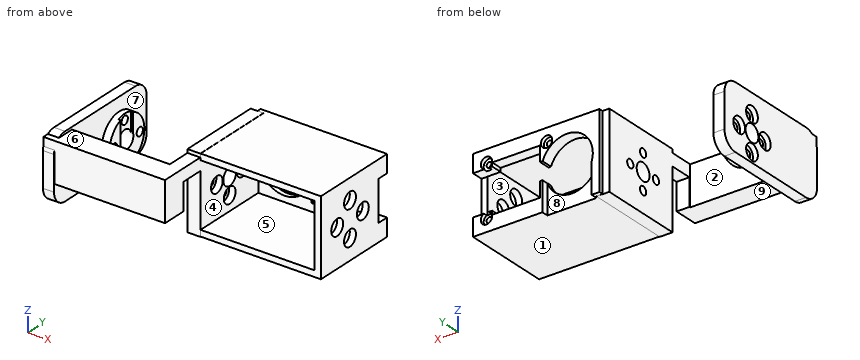
from build123d import *

# Parameters (mm, degrees)
S_PRISM1_W      = 30.9
S_PRISM1_H      = 34.5
BOSS_1_DEPTH    = 5.2
S_CYL2_R        = 9.5
BOSS_2_DEPTH    = 3.2
BOSS_3_DEPTH    = 4.5
S_BOX4_W        = 2.5
S_BOX4_H        = 36.1
BOSS_4_DEPTH    = 30.8
S_BOX5_W        = 2.5
S_BOX5_H        = 36.1
BOSS_5_DEPTH    = 30.8
S_BOX6_W        = 51.4
S_BOX6_H        = 36.1
BOSS_6_DEPTH    = 2.5
S_BOX7_W        = 51.4
S_BOX7_H        = 36.1
BOSS_7_DEPTH    = 2.5
S_BOX8_W        = 51.4
S_BOX8_H        = 4.6
BOSS_8_DEPTH    = 30.8
S_BOX9_W        = 5.2
S_BOX9_H        = 9.8
BOSS_9_DEPTH    = 5
S_BOX10_W       = 5.2
S_BOX10_H       = 10
BOSS_10_DEPTH   = 16
S_BOX11_W       = 49.45
S_BOX11_H       = 9.6
BOSS_11_DEPTH   = 16
S_HOLE12_R      = 3.5
HOLE_12_DEPTH   = 5.4
S_HOLE13_R      = 1.7
HOLE_13_DEPTH   = 5.4
S_HOLE14_R      = 1.7
HOLE_14_DEPTH   = 5.4
S_HOLE15_R      = 1.7
HOLE_15_DEPTH   = 5.4
S_HOLE16_R      = 1.7
HOLE_16_DEPTH   = 5.4
S_HOLE17_R      = 3.2
HOLE_17_DEPTH   = 2.7
S_HOLE18_R      = 3.2
HOLE_18_DEPTH   = 2.7
S_HOLE19_R      = 3.2
HOLE_19_DEPTH   = 2.7
S_HOLE20_R      = 3.2
HOLE_20_DEPTH   = 2.7
S_HOLE21_R      = 3.5
HOLE_21_DEPTH   = 7.9
S_HOLE22_R      = 1.7
HOLE_22_DEPTH   = 7.9
S_HOLE23_R      = 1.7
HOLE_23_DEPTH   = 7.9
S_HOLE24_R      = 1.7
HOLE_24_DEPTH   = 7.9
S_HOLE25_R      = 1.7
HOLE_25_DEPTH   = 7.9
S_HOLE26_R      = 3.2
HOLE_26_DEPTH   = 2.1
S_HOLE27_R      = 3.2
HOLE_27_DEPTH   = 2.1
S_HOLE28_R      = 3.2
HOLE_28_DEPTH   = 2.1
S_HOLE29_R      = 3.2
HOLE_29_DEPTH   = 2.1
S_CUT30_W       = 1
S_CUT30_H       = 6.8
POCKET_30_DEPTH = 10
S_HOLE31_R      = 10.5
HOLE_31_DEPTH   = 4.8
S_CUT32_W       = 19.5
S_CUT32_H       = 4.75
POCKET_32_DEPTH = 19.4
S_CUT33_W       = 8.3
S_CUT33_H       = 4.75
POCKET_33_DEPTH = 16.4
S_CUT34_W       = 11
S_CUT34_H       = 4.75
POCKET_34_DEPTH = 7
S_CUT35_W       = 20
S_CUT35_H       = 2.9
POCKET_35_DEPTH = 15.9
S_HOLE36_R      = 1.1
HOLE_36_DEPTH   = 4.8
S_HOLE37_R      = 2.3
HOLE_37_DEPTH   = 1.7
S_HOLE38_R      = 1.1
HOLE_38_DEPTH   = 4.8
S_HOLE39_R      = 2.3
HOLE_39_DEPTH   = 1.7
S_HOLE40_R      = 1.1
HOLE_40_DEPTH   = 4.8
S_HOLE41_R      = 2.3
HOLE_41_DEPTH   = 1.7
S_HOLE42_R      = 3.25
HOLE_42_DEPTH   = 2.7
S_HOLE43_R      = 3.25
HOLE_43_DEPTH   = 2.7
S_HOLE44_R      = 3.25
HOLE_44_DEPTH   = 2.7
S_HOLE45_R      = 3.25
HOLE_45_DEPTH   = 2.7


with BuildPart() as part:
    # S_prism1 → Boss_1 (new body)
    with BuildSketch(Plane(origin=(-15.9, 0, 0), x_dir=(0, 0, -1), z_dir=(1, 0, 0))):
        with Locations((0, 1.2)):
            Rectangle(S_PRISM1_W, S_PRISM1_H)
    extrude(amount=BOSS_1_DEPTH)

    # S_box4 → Boss_4 (add)
    with BuildSketch(Plane.XY.offset(-15.4)):
        with Locations((-11.95, 2.15)):
            Rectangle(S_BOX4_W, S_BOX4_H)
    extrude(amount=BOSS_4_DEPTH)



with BuildPart() as body_2:
    # S_cyl2 → Boss_2 (new body)
    with BuildSketch(Plane(origin=(-55.65, 0, 0), x_dir=(0, 0, -1), z_dir=(1, 0, 0))):
        Circle(S_CYL2_R)
    extrude(amount=BOSS_2_DEPTH)

    # S_prism3 → Boss_3 (add)
    with BuildSketch(Plane(origin=(-60.15, 0, 0), x_dir=(0, 0, -1), z_dir=(1, 0, 0))):
        with BuildLine():
            Line((11, 9), (11, -29.5))
            ThreePointArc((11, -29.5), (9.2426, -33.7426), (5, -35.5))
            Line((5, -35.5), (-9, -35.5))
            ThreePointArc((-9, -35.5), (-13.2426, -33.7426), (-15, -29.5))
            Line((-15, -29.5), (-15, 9))
            ThreePointArc((-15, 9), (-13.2426, 13.2426), (-9, 15))
            Line((-9, 15), (5, 15))
            ThreePointArc((5, 15), (9.2426, 13.2426), (11, 9))
        make_face()
    extrude(amount=BOSS_3_DEPTH)


with BuildPart() as body_3:
    # S_box5 → Boss_5 (new body)
    with BuildSketch(Plane.XY.offset(-15.4)):
        with Locations((36.95, 2.15)):
            Rectangle(S_BOX5_W, S_BOX5_H)
    extrude(amount=BOSS_5_DEPTH)


with BuildPart() as part_1:
    add(part.part)

    add(body_3.part)  # Boss_6 merges body 3
    # S_box6 → Boss_6 (add)
    with BuildSketch(Plane.XY.offset(-15.4)):
        with Locations((12.5, 2.15)):
            Rectangle(S_BOX6_W, S_BOX6_H)
    extrude(amount=BOSS_6_DEPTH)

    # S_box7 → Boss_7 (add)
    with BuildSketch(Plane.XY.offset(12.9)):
        with Locations((12.5, 2.15)):
            Rectangle(S_BOX7_W, S_BOX7_H)
    extrude(amount=BOSS_7_DEPTH)

    # S_box8 → Boss_8 (add)
    with BuildSketch(Plane.XY.offset(-15.4)):
        with Locations((12.5, 17.9)):
            Rectangle(S_BOX8_W, S_BOX8_H)
    extrude(amount=BOSS_8_DEPTH)

    # S_box9 → Boss_9 (add)
    with BuildSketch(Plane.XY.offset(9)):
        with Locations((-13.3, -20.9)):
            Rectangle(S_BOX9_W, S_BOX9_H)
    extrude(amount=BOSS_9_DEPTH)

    # S_box10 → Boss_10 (add)
    with BuildSketch(Plane.XY.offset(-2)):
        with Locations((-13.3, -30.3)):
            Rectangle(S_BOX10_W, S_BOX10_H)
    extrude(amount=BOSS_10_DEPTH)


    add(body_2.part)  # Boss_11 merges body 2
    # S_box11 → Boss_11 (add)
    with BuildSketch(Plane.XY.offset(-2)):
        with Locations((-35.425, -30.5)):
            Rectangle(S_BOX11_W, S_BOX11_H)
    extrude(amount=BOSS_11_DEPTH)

    # S_hole12 → Hole_12 (cut)
    with BuildSketch(Plane(origin=(-16, 0, 0), x_dir=(0, 0, -1), z_dir=(1, 0, 0))):
        with Locations(Location((0, 0, 0), (0, 0, 180))):
            Circle(S_HOLE12_R)
    extrude(amount=HOLE_12_DEPTH, mode=Mode.SUBTRACT)

    # S_hole13 → Hole_13 (cut)
    with BuildSketch(Plane(origin=(-16, 0, 0), x_dir=(0, 0, -1), z_dir=(1, 0, 0))):
        with Locations(Location((0, -7, 0), (0, 0, 180))):
            Circle(S_HOLE13_R)
    extrude(amount=HOLE_13_DEPTH, mode=Mode.SUBTRACT)

    # S_hole14 → Hole_14 (cut)
    with BuildSketch(Plane(origin=(-16, 0, 0), x_dir=(0, 0, -1), z_dir=(1, 0, 0))):
        with Locations(Location((-7, 0, 0), (0, 0, 180))):
            Circle(S_HOLE14_R)
    extrude(amount=HOLE_14_DEPTH, mode=Mode.SUBTRACT)

    # S_hole15 → Hole_15 (cut)
    with BuildSketch(Plane(origin=(-16, 0, 0), x_dir=(0, 0, -1), z_dir=(1, 0, 0))):
        with Locations(Location((0, 7, 0), (0, 0, 180))):
            Circle(S_HOLE15_R)
    extrude(amount=HOLE_15_DEPTH, mode=Mode.SUBTRACT)

    # S_hole16 → Hole_16 (cut)
    with BuildSketch(Plane(origin=(-16, 0, 0), x_dir=(0, 0, -1), z_dir=(1, 0, 0))):
        with Locations(Location((7, 0, 0), (0, 0, 180))):
            Circle(S_HOLE16_R)
    extrude(amount=HOLE_16_DEPTH, mode=Mode.SUBTRACT)

    # S_hole17 → Hole_17 (cut)
    with BuildSketch(Plane(origin=(-13.3, 0, 0), x_dir=(0, 0, -1), z_dir=(1, 0, 0))):
        with Locations(Location((0, -7, 0), (0, 0, 180))):
            Circle(S_HOLE17_R)
    extrude(amount=HOLE_17_DEPTH, mode=Mode.SUBTRACT)

    # S_hole18 → Hole_18 (cut)
    with BuildSketch(Plane(origin=(-13.3, 0, 0), x_dir=(0, 0, -1), z_dir=(1, 0, 0))):
        with Locations(Location((-7, 0, 0), (0, 0, 180))):
            Circle(S_HOLE18_R)
    extrude(amount=HOLE_18_DEPTH, mode=Mode.SUBTRACT)

    # S_hole19 → Hole_19 (cut)
    with BuildSketch(Plane(origin=(-13.3, 0, 0), x_dir=(0, 0, -1), z_dir=(1, 0, 0))):
        with Locations(Location((0, 7, 0), (0, 0, 180))):
            Circle(S_HOLE19_R)
    extrude(amount=HOLE_19_DEPTH, mode=Mode.SUBTRACT)

    # S_hole20 → Hole_20 (cut)
    with BuildSketch(Plane(origin=(-13.3, 0, 0), x_dir=(0, 0, -1), z_dir=(1, 0, 0))):
        with Locations(Location((7, 0, 0), (0, 0, 180))):
            Circle(S_HOLE20_R)
    extrude(amount=HOLE_20_DEPTH, mode=Mode.SUBTRACT)

    # S_hole21 → Hole_21 (cut)
    with BuildSketch(Plane(origin=(-60.25, 0, 0), x_dir=(0, 0, -1), z_dir=(1, 0, 0))):
        with Locations(Location((0, 0, 0), (0, 0, 180))):
            Circle(S_HOLE21_R)
    extrude(amount=HOLE_21_DEPTH, mode=Mode.SUBTRACT)

    # S_hole22 → Hole_22 (cut)
    with BuildSketch(Plane(origin=(-60.25, 0, 0), x_dir=(0, 0, -1), z_dir=(1, 0, 0))):
        with Locations(Location((0, -7, 0), (0, 0, 180))):
            Circle(S_HOLE22_R)
    extrude(amount=HOLE_22_DEPTH, mode=Mode.SUBTRACT)

    # S_hole23 → Hole_23 (cut)
    with BuildSketch(Plane(origin=(-60.25, 0, 0), x_dir=(0, 0, -1), z_dir=(1, 0, 0))):
        with Locations(Location((-7, 0, 0), (0, 0, 180))):
            Circle(S_HOLE23_R)
    extrude(amount=HOLE_23_DEPTH, mode=Mode.SUBTRACT)

    # S_hole24 → Hole_24 (cut)
    with BuildSketch(Plane(origin=(-60.25, 0, 0), x_dir=(0, 0, -1), z_dir=(1, 0, 0))):
        with Locations(Location((0, 7, 0), (0, 0, 180))):
            Circle(S_HOLE24_R)
    extrude(amount=HOLE_24_DEPTH, mode=Mode.SUBTRACT)

    # S_hole25 → Hole_25 (cut)
    with BuildSketch(Plane(origin=(-60.25, 0, 0), x_dir=(0, 0, -1), z_dir=(1, 0, 0))):
        with Locations(Location((7, 0, 0), (0, 0, 180))):
            Circle(S_HOLE25_R)
    extrude(amount=HOLE_25_DEPTH, mode=Mode.SUBTRACT)

    # S_hole26 → Hole_26 (cut)
    with BuildSketch(Plane(origin=(-60.25, 0, 0), x_dir=(0, 0, -1), z_dir=(1, 0, 0))):
        with Locations(Location((0, -7, 0), (0, 0, 180))):
            Circle(S_HOLE26_R)
    extrude(amount=HOLE_26_DEPTH, mode=Mode.SUBTRACT)

    # S_hole27 → Hole_27 (cut)
    with BuildSketch(Plane(origin=(-60.25, 0, 0), x_dir=(0, 0, -1), z_dir=(1, 0, 0))):
        with Locations(Location((-7, 0, 0), (0, 0, 180))):
            Circle(S_HOLE27_R)
    extrude(amount=HOLE_27_DEPTH, mode=Mode.SUBTRACT)

    # S_hole28 → Hole_28 (cut)
    with BuildSketch(Plane(origin=(-60.25, 0, 0), x_dir=(0, 0, -1), z_dir=(1, 0, 0))):
        with Locations(Location((0, 7, 0), (0, 0, 180))):
            Circle(S_HOLE28_R)
    extrude(amount=HOLE_28_DEPTH, mode=Mode.SUBTRACT)

    # S_hole29 → Hole_29 (cut)
    with BuildSketch(Plane(origin=(-60.25, 0, 0), x_dir=(0, 0, -1), z_dir=(1, 0, 0))):
        with Locations(Location((7, 0, 0), (0, 0, 180))):
            Circle(S_HOLE29_R)
    extrude(amount=HOLE_29_DEPTH, mode=Mode.SUBTRACT)

    # S_cut30 → Pocket_30 (cut)
    with BuildSketch(Plane.XY):
        with Locations((-52.85, 0)):
            Rectangle(S_CUT30_W, S_CUT30_H)
    extrude(amount=POCKET_30_DEPTH, mode=Mode.SUBTRACT)

    # S_hole31 → Hole_31 (cut)
    with BuildSketch(Plane(origin=(0, 15.5, 0), x_dir=(1, 0, 0), z_dir=(0, 1, 0))):
        with Locations(Location((0, 0, 0), (0, 0, 90))):
            Circle(S_HOLE31_R)
    extrude(amount=HOLE_31_DEPTH, mode=Mode.SUBTRACT)

    # S_cut32 → Pocket_32 (cut)
    with BuildSketch(Plane.XY.offset(-9.7)):
        with Locations((20.65, 17.925)):
            Rectangle(S_CUT32_W, S_CUT32_H)
    extrude(amount=POCKET_32_DEPTH, mode=Mode.SUBTRACT)

    # S_cut33 → Pocket_33 (cut)
    with BuildSketch(Plane.XY.offset(-8.2)):
        with Locations((34.55, 17.925)):
            Rectangle(S_CUT33_W, S_CUT33_H)
    extrude(amount=POCKET_33_DEPTH, mode=Mode.SUBTRACT)

    # S_cut34 → Pocket_34 (cut)
    with BuildSketch(Plane.XY.offset(-3.5)):
        with Locations((5.5, 17.925)):
            Rectangle(S_CUT34_W, S_CUT34_H)
    extrude(amount=POCKET_34_DEPTH, mode=Mode.SUBTRACT)

    # S_cut35 → Pocket_35 (cut)
    with BuildSketch(Plane.XY.offset(-15.9)):
        with Locations((0, 18.95)):
            Rectangle(S_CUT35_W, S_CUT35_H)
    extrude(amount=POCKET_35_DEPTH, mode=Mode.SUBTRACT)

    # S_hole36 → Hole_36 (cut)
    with BuildSketch(Plane(origin=(0, 15.5, 0), x_dir=(1, 0, 0), z_dir=(0, 1, 0))):
        with Locations(Location((8.3, -10.25, 0), (0, 0, 90))):
            Circle(S_HOLE36_R)
    extrude(amount=HOLE_36_DEPTH, mode=Mode.SUBTRACT)

    # S_hole37 → Hole_37 (cut)
    with BuildSketch(Plane(origin=(0, 18.6, 0), x_dir=(1, 0, 0), z_dir=(0, 1, 0))):
        with Locations(Location((8.3, -10.25, 0), (0, 0, 90))):
            Circle(S_HOLE37_R)
    extrude(amount=HOLE_37_DEPTH, mode=Mode.SUBTRACT)

    # S_hole38 → Hole_38 (cut)
    with BuildSketch(Plane(origin=(0, 15.5, 0), x_dir=(1, 0, 0), z_dir=(0, 1, 0))):
        with Locations(Location((32.75, 10.25, 0), (0, 0, 90))):
            Circle(S_HOLE38_R)
    extrude(amount=HOLE_38_DEPTH, mode=Mode.SUBTRACT)

    # S_hole39 → Hole_39 (cut)
    with BuildSketch(Plane(origin=(0, 18.6, 0), x_dir=(1, 0, 0), z_dir=(0, 1, 0))):
        with Locations((32.75, 10.25)):
            Circle(S_HOLE39_R)
    extrude(amount=HOLE_39_DEPTH, mode=Mode.SUBTRACT)

    # S_hole40 → Hole_40 (cut)
    with BuildSketch(Plane(origin=(0, 15.5, 0), x_dir=(1, 0, 0), z_dir=(0, 1, 0))):
        with Locations(Location((32.75, -10.25, 0), (0, 0, 90))):
            Circle(S_HOLE40_R)
    extrude(amount=HOLE_40_DEPTH, mode=Mode.SUBTRACT)

    # S_hole41 → Hole_41 (cut)
    with BuildSketch(Plane(origin=(0, 18.6, 0), x_dir=(1, 0, 0), z_dir=(0, 1, 0))):
        with Locations((32.75, -10.25)):
            Circle(S_HOLE41_R)
    extrude(amount=HOLE_41_DEPTH, mode=Mode.SUBTRACT)

    # S_hole42 → Hole_42 (cut)
    with BuildSketch(Plane(origin=(35.6, 0, 0), x_dir=(0, 0, -1), z_dir=(1, 0, 0))):
        with Locations(Location((0, -7, 0), (0, 0, 180))):
            Circle(S_HOLE42_R)
    extrude(amount=HOLE_42_DEPTH, mode=Mode.SUBTRACT)

    # S_hole43 → Hole_43 (cut)
    with BuildSketch(Plane(origin=(35.6, 0, 0), x_dir=(0, 0, -1), z_dir=(1, 0, 0))):
        with Locations(Location((-7, 0, 0), (0, 0, 180))):
            Circle(S_HOLE43_R)
    extrude(amount=HOLE_43_DEPTH, mode=Mode.SUBTRACT)

    # S_hole44 → Hole_44 (cut)
    with BuildSketch(Plane(origin=(35.6, 0, 0), x_dir=(0, 0, -1), z_dir=(1, 0, 0))):
        with Locations(Location((0, 7, 0), (0, 0, 180))):
            Circle(S_HOLE44_R)
    extrude(amount=HOLE_44_DEPTH, mode=Mode.SUBTRACT)

    # S_hole45 → Hole_45 (cut)
    with BuildSketch(Plane(origin=(35.6, 0, 0), x_dir=(0, 0, -1), z_dir=(1, 0, 0))):
        with Locations(Location((7, 0, 0), (0, 0, 180))):
            Circle(S_HOLE45_R)
    extrude(amount=HOLE_45_DEPTH, mode=Mode.SUBTRACT)


solid = part_1.part
Source: CAD feature listing. Evaluate the final solid. Frame: model axes, mm. Face numbers are marked on the shaded views. A direction names the side the tool comes from. Coordinates: 2 decimals unless noted, no trailing zeros. Order: outer loops, then holes, each group sorted by start corner. A loop starts at its lowest first (then second) coordinate and runs counter-clockwise, first axis right, second up. Notation, with made-up numbers: M 44.25,0.5 L 65.25,0.5 A21 ccw 65.25,22.5 Z; hole C -1.75,-34.5 d7. An arc over 180 degrees is marked long. Write each question's results on one line, items separated by ' | '. Start each with the question number.
Item 1: Cut plane B-B (y = -21). Return loops of the section in (x, z), and give its area (3 significant figures).
Item 2: Set-up query: the marked faces 5, 6, 7, 8 and 9. Return all of +Z, -Z, +X, -X, +Y, -Y with unobstructed straight access to the full face (end or side cutting, diameter ignored); none if empty.
Item 3: Cut plane D-D (y = 0). Count the separate pieces of the cut face and the enclosed holes in it, and give its area (3 significant figures).
Item 4: Cut plane A-A (x = 23). Return loops of the section in (y, z).
Item 5: First-contact query: pin 1 Ø4 at (x, y) = (-13, -21.5) entering from -Z; pin 2 Ø5 at (x, y) = (32.5, 17.5) entering from -Z; pin 3 Ø5 at (x, y) = (-11, -24.5) entering from +Z; pin 4 Ø2 at (y, z) = (0, -7) entering from -X. Flat tips, straight axial feed; report the tip coordinate or a pass-through.
Item 6: Cut plane C-C (x = 0). Return loops of the section in (y, z).
Item 7: Line query: probe 1 along X at (y, z) = (-3.5, -7.5); probe 2 along X at (y, z) = (-7.5, 11.5); probe 3 along X at (y, z) = (-21.5, 12). Output: solid intervals per line, ascending.
Item 8: Draft query along Z for the marked faces 1, 2, 3 and 4. Return one class per face: pulls with the +Z half, pulls with the -Z half, needs draft (parallel to the pull), parting line crosses it, or undercut.
Checked values:
1) outline: M -60.15,-11 L -55.65,-11 L -55.65,15 L -60.15,15 Z; M -15.9,9 L -10.7,9 L -10.7,14 L -15.9,14 Z | area: 143 mm2
2) face 5: -Y | face 6: +Z, +X, -Y | face 7: none | face 8: -Z, +Y | face 9: -Z, +X, -Y
3) separate pieces: 9 | enclosed holes: 0 | area: 407 mm2
4) outline: M -15.9,-15.4 L 20.2,-15.4 L 20.2,-9.7 L 15.6,-9.7 L 15.6,-12.9 L -15.9,-12.9 Z; M -15.9,12.9 L 15.6,12.9 L 15.6,9.7 L 20.2,9.7 L 20.2,15.4 L -15.9,15.4 Z
5) pin 1: stops at z = 9 | pin 2: stops at z = -15.4 | pin 3: stops at z = 14 | pin 4: passes through
6) outline: M -15.9,-15.4 L 17.5,-15.4 L 17.5,-10.5 L 15.6,-10.5 L 15.6,-12.9 L -15.9,-12.9 Z; M -15.9,12.9 L 15.6,12.9 L 15.6,10.5 L 20.2,10.5 L 20.2,15.4 L -15.9,15.4 Z
7) probe 1: x = -60.15 to -52.45, -15.9 to -10.7, 35.7 to 38.2 | probe 2: x = -60.15 to -55.65, -15.9 to -10.7, 35.7 to 38.2 | probe 3: x = -60.15 to -55.65, -15.9 to -10.7
8) face 1: pulls with the -Z half | face 2: needs draft | face 3: undercut | face 4: undercut
